from build123d import *

# Parameters (mm, degrees)
F0_W      = 22.86
F0_H      = 10.16
F1_DEPTH  = 25
F2_W      = 7.1686236836
F2_H      = 5.1849592477
F3_DEPTH  = 5
F4_W      = 9.9097841885
F4_H      = 8.9319869876
F5_DEPTH  = 3
F6_W      = 10.2559335064
F6_H      = 16.0680130124
F7_DEPTH  = 6
F8_W      = 3.1437913674
F8_H      = 8.0340065062
F9_DEPTH  = 25
F10_W     = 8.0340065062
F10_H     = 6
F11_DEPTH = 7.2244124593
F12_W     = 7.2234124593
F12_H     = 8.0340065062
F13_DEPTH = 2
F14_DEPTH = 5.7


# Not quite as in the source:
# - a feature names something its author has since deleted; it is built from what else it names


with BuildPart() as f1:
    # F0 (on Front) → F1 (new body)
    with BuildSketch(Plane.XZ):
        with Locations((0.6582729786, 5.08)):
            Rectangle(F0_W, F0_H)
    extrude(amount=F1_DEPTH)

    # F2 (on face) → F3 (cut)
    with BuildSketch(Plane.XY.offset(10.16)):
        with Locations((-7.1874151796, -22.4075203761)):
            Rectangle(F2_W, F2_H)
    extrude(amount=-F3_DEPTH, mode=Mode.SUBTRACT)

    # F4 (on face) → F5 (cut)
    with BuildSketch(Plane.XY.offset(10.16)):
        with Locations((1.4065775322, -4.4659934938)):
            Rectangle(F4_W, F4_H)
    extrude(amount=-F5_DEPTH, mode=Mode.SUBTRACT)

    # F6 (on face) → F7 (cut)
    with BuildSketch(Plane.XY.offset(10.16)):
        with Locations((1.5796521911, -16.9659934938)):
            Rectangle(F6_W, F6_H)
        Polygon((6.3614696264, 0), (6.3614696264, -8.9319869876), (6.7076189443, -8.9319869876), (6.7076189443, -25), (12.0882729786, -25), (12.0882729786, 0), align=None)
    extrude(amount=-F7_DEPTH, mode=Mode.SUBTRACT)

    # F8 (on face) → F9 (cut)
    with BuildSketch(Plane.XY.offset(4.16)):
        with Locations((10.5163772949, -20.9829967469)):
            Rectangle(F8_W, F8_H)
    extrude(amount=-F9_DEPTH, mode=Mode.SUBTRACT)

    # F10 (on face) → F11 (cut, through all)
    with BuildSketch(Plane.YZ.offset(-3.5483145621)):
        with Locations((-20.9829967469, 7.16)):
            Rectangle(F10_W, F10_H)
    extrude(amount=-F11_DEPTH, mode=Mode.SUBTRACT)

    # F12 (on face) → F13 (join)
    with BuildSketch(Plane.XY.offset(4.16)):
        with Locations((-7.1600207917, -20.9829967469)):
            Rectangle(F12_W, F12_H)
    extrude(amount=F13_DEPTH)

    # F14 (add): a face of the model
    f14_faces = [f1.faces().sort_by_distance(p)[0] for p in [
        (12.0882729786, -8.4829967469, 2.08),
    ]]
    extrude(f14_faces, amount=F14_DEPTH)


solid = f1.part
Part model, mm, in its own coordinate system. A direction names the side the tool comes from. Give positions to 0.01 mm unless a question says otherwise; leave off trailing zeros. Loops run counter-clockwise (first coordinate to the right, second up) from the corner with the lowest first, then second, coordinate; pieces in that order, holes last.
(1) Band-saw the part on B-B (z = 4.5). Write the cut outline in (x, y), and give its area (3 significant figures).
Return value:
outline: (-10.77, -25) - (-3.55, -25) - (-3.55, -8.93) - (6.36, -8.93) - (6.36, 0) - (-10.77, 0) - close
area: 269 mm2
(2) Drill centre lines: line 1 along Z through (x, y) = (-4.5, -22.5); line 2 along Z through (x, y) = (2.25, -22.5); line 3 along Y through (x, z) = (14.5, 4). Where is each one in solid material? Low to high.
Return value:
line 1: z = 0 to 6.16
line 2: z = 0 to 4.16
line 3: y = -16.97 to 0
(3) Band-saw the part on A-A (y = -3.5). Write the cut outline in (x, z), and give its area (3 significant figures).
Return value:
outline: (-10.77, 0) - (17.79, 0) - (17.79, 4.16) - (6.36, 4.16) - (6.36, 7.16) - (-3.55, 7.16) - (-3.55, 10.16) - (-10.77, 10.16) - close
area: 192 mm2
(4) Pin check, flat tips, straight feed: pin 1 (3.5 mm diameter, centred on y = -4, z = 6, fed in from +X); pin 2 (4.5 mm diameter, centred on x = 12.5, z = 2.5, fed in from -Y); pin 3 (1.8 mm diameter, centred on y = -7.5, z = 8.5, fed in from +X). Stop position of each tip, or through.
Return value:
pin 1: stops at x = 6.36
pin 2: stops at y = -16.97
pin 3: stops at x = -3.55
(5) Band-saw the part on D-D (z = 9.25). Write the cut outline in (x, y), and give its area (3 significant figures).
Return value:
outline: (-10.77, -16.97) - (-3.55, -16.97) - (-3.55, 0) - (-10.77, 0) - close
area: 123 mm2
(6) Band-saw the part on C-C (x = 0.5). Write the cut outline in (y, z).
Return value:
outline: (-25, 0) - (0, 0) - (0, 7.16) - (-8.93, 7.16) - (-8.93, 4.16) - (-25, 4.16) - close
(7) 3-axis set-ups, long thin cutter, end or side, ignore diameter. For faces 1 (the flat face through (1, -4, 7.16)), 2 (the flat face through (13, -16.966, 2)), 3 (the flat face through (1, -8.932, 6)), 4 (the flat face through (-7, -21, 6.16)): which of +Z, -Z, +X, -X, +Y, -Y reach the whole face in a straight line?
Return value:
face 1: +Z, +X, +Y, -Y
face 2: +Z, -Z, +X, -Y
face 3: +Z, +X, -Y
face 4: +Z, +X, -X, -Y
